from build123d import *

# Parameters (mm, degrees)
F0_R     = 2.286
F0_R_2   = 7.9375
F1_DEPTH = 3.81


with BuildPart() as f1:
    # F0 (on Top) → F1 (new body)
    with BuildSketch(Plane.XY):
        with BuildLine():
            Line((2.435129, 67.945), (-2.435129, 67.945))
            ThreePointArc((-2.435129, 67.945), (-3.826344, 68.359884), (-4.763077, 69.469))
            ThreePointArc((-4.763077, 69.469), (-10.056534, 71.302168), (-11.4554, 65.877746))
            ThreePointArc((-11.4554, 65.877746), (-11.152718, 65.217997), (-11.049, 64.499576))
            Line((-11.049, 64.499576), (-11.049, -62.125129))
            ThreePointArc((-11.049, -62.125129), (-11.463884, -63.516344), (-12.573, -64.453077))
            ThreePointArc((-12.573, -64.453077), (-13.743077, -70.639077), (-7.557077, -69.469))
            ThreePointArc((-7.557077, -69.469), (-6.620344, -68.359884), (-5.229129, -67.945))
            Line((-5.229129, -67.945), (5.229129, -67.945))
            ThreePointArc((5.229129, -67.945), (6.620344, -68.359884), (7.557077, -69.469))
            ThreePointArc((7.557077, -69.469), (13.743077, -70.639077), (12.573, -64.453077))
            ThreePointArc((12.573, -64.453077), (11.463884, -63.516344), (11.049, -62.125129))
            Line((11.049, -62.125129), (11.049, 64.499576))
            ThreePointArc((11.049, 64.499576), (11.152718, 65.217997), (11.4554, 65.877746))
            ThreePointArc((11.4554, 65.877746), (10.056534, 71.302168), (4.763077, 69.469))
            ThreePointArc((4.763077, 69.469), (3.826344, 68.359884), (2.435129, 67.945))
        make_face()
        with Locations((-11.049, -67.945)):
            Circle(F0_R, mode=Mode.SUBTRACT)
        with Locations((0, -50.8)):
            Circle(F0_R_2, mode=Mode.SUBTRACT)
        with Locations((0, -25.4)):
            Circle(F0_R_2, mode=Mode.SUBTRACT)
        with Locations((11.049, -67.945)):
            Circle(F0_R, mode=Mode.SUBTRACT)
        Circle(F0_R_2, mode=Mode.SUBTRACT)
        with Locations((0, 25.4)):
            Circle(F0_R_2, mode=Mode.SUBTRACT)
        with Locations((-8.255, 67.945)):
            Circle(F0_R, mode=Mode.SUBTRACT)
        with Locations((0, 50.8)):
            Circle(F0_R_2, mode=Mode.SUBTRACT)
        with Locations((8.255, 67.945)):
            Circle(F0_R, mode=Mode.SUBTRACT)
    extrude(amount=F1_DEPTH)


solid = f1.part
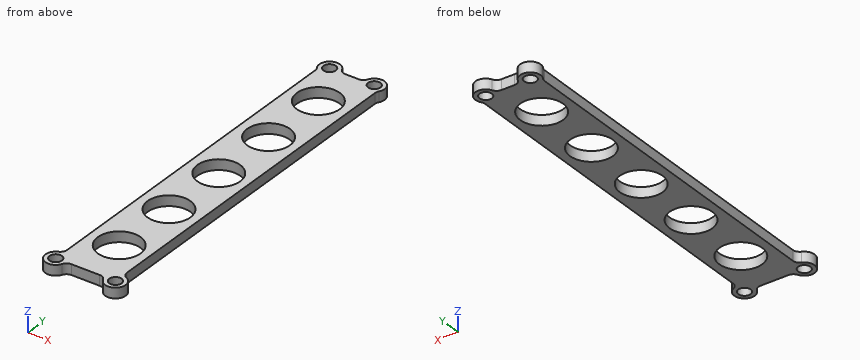
Design review of the part built by this model. Coordinates are the model's own, in mm. Give positions to 0.01 mm unless a question says otherwise; leave off trailing zeros. Write each loop counter-clockwise with the first axis right and the second up, starting at its lowest first coordinate (ties: lowest second). Pieces come first, ordered by that corner, then holes. Notation, with made-up numbers: M 69.25,88.25 L 89.25,88.25 A19 cw 89.25,102.25 Z; hole C 82,67 d8. An arc over 180 degrees is marked long. Return JSON: item names as keys, results as strings. Group by question number.
Item 1: Clearance check with flat-ended pins moving along their axes: pin 1 Ø12 at (x, y) = (-3, -55) entering from +Z; pin 2 Ø2 at (x, z) = (2, 1) entering from -Y (3 decimals); pin 3 Ø1.1 at (y, z) = (3.5, 2.5) entering from -X; pin 4 Ø1 at (x, z) = (5, 0.5) entering from -Y. State where each tip first meets the part, or that it passes through.
Item 2: Take a section at A-A (z = 0.95). Count the separate pieces of the cut face and the enclosed holes in it, plus the area to 3 significant figures.
Item 3: Take a section at C-C (x = -0.5). Give the boundary of the cut face in (y, z) (3 decimals).
Item 4: Take a section at B-B (y = -50.8). Give the boundary of the cut face in (x, z), plus the area to 3 significant figures.
Item 5: Wall thickness on line 1 along Y through (x, z) = (0, 0.8) (1 decimal); line 2 along X through (y, z) = (-23, 2); line 3 along Y through (x, z) = (-4.5, 0.9) (3 decimals): over which ranges is each line inside the solid? List them lowest first.
Item 6: Take a section at D-D (y = 14.5). Give the boundary of the cut face in (x, z).
Return value:
{
 "1": {"pin 1": "stops at z = 3.81", "pin 2": "stops at y = -67.945", "pin 3": "stops at x = -11.05", "pin 4": "stops at y = -67.96"},
 "2": {"separate pieces": "1", "enclosed holes": "9", "area": "2,070 mm2"},
 "3": {"outline": "M -67.945,0 L -58.722,0 L -58.722,3.81 L -67.945,3.81 Z; M -42.878,0 L -33.322,0 L -33.322,3.81 L -42.878,3.81 Z; M -17.478,0 L -7.922,0 L -7.922,3.81 L -17.478,3.81 Z; M 7.922,0 L 17.478,0 L 17.478,3.81 L 7.922,3.81 Z; M 33.322,0 L 42.878,0 L 42.878,3.81 L 33.322,3.81 Z; M 58.722,0 L 67.945,0 L 67.945,3.81 L 58.722,3.81 Z"},
 "4": {"outline": "M -11.05,0 L -7.94,0 L -7.94,3.81 L -11.05,3.81 Z; M 7.94,0 L 11.05,0 L 11.05,3.81 L 7.94,3.81 Z", "area": "23.7 mm2"},
 "5": {"line 1": "y = -67.9 to -58.7, -42.9 to -33.3, -17.5 to -7.9, 7.9 to 17.5, 33.3 to 42.9, 58.7 to 67.9", "line 2": "x = -11.05 to -7.57, 7.57 to 11.05", "line 3": "y = -67.945 to -57.339, -44.261 to -31.939, -18.861 to -6.539, 6.539 to 18.861, 31.939 to 44.261, 57.339 to 69.006"},
 "6": {"outline": "M -11.05,0 L 11.05,0 L 11.05,3.81 L -11.05,3.81 Z"}
}
